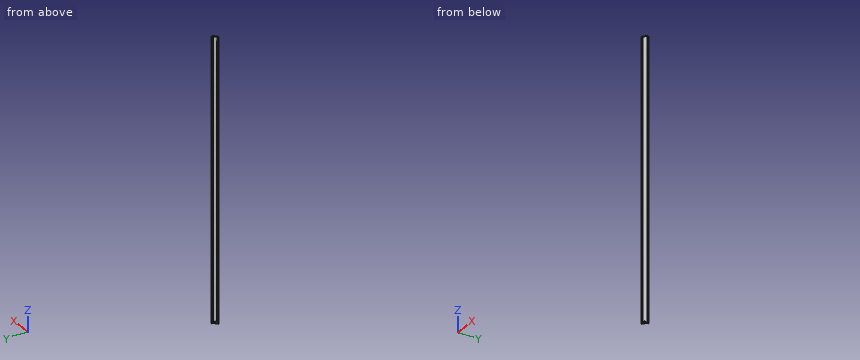
from build123d import *

# Parameters (mm, degrees)
F1_DEPTH = 28
F3_DEPTH = 2653
F5_DEPTH = 28
F6_R     = 2
F7_R     = 1
F8_R     = 4.25
F9_DEPTH = 25


with BuildPart() as f1:
    # F0 (on Top) → F1 (new body)
    with BuildSketch(Plane.XY):
        Polygon((-19.75, -17.750001), (-19.75, -19.75), (-9.25, -19.75), (19.75, 9.25), (19.75, 19.75), (17.750001, 19.75), (17.750001, 10.078427), (-10.078427, -17.750001), align=None)
    extrude(amount=F1_DEPTH)

    # F2 (on face) → F3 (join)
    with BuildSketch(Plane.XY.offset(28)):
        Polygon((-19.75, -19.75), (-9.25, -19.75), (19.75, 9.25), (19.75, 19.75), (11.25, 19.75), (11.25, 24.25), (9.25, 26.25), (9.25, 23.421573), (9.25, 19.75), (9.25, 17.750001), (17.750001, 17.750001), (17.750001, 10.078427), (16.585787, 8.914213), (-8.914213, -16.585787), (-10.078427, -17.750001), (-17.750001, -17.750001), (-17.750001, -9.25), (-19.75, -9.25), (-23.421573, -9.25), (-26.25, -9.25), (-24.25, -11.25), (-19.75, -11.25), align=None)
    extrude(amount=F3_DEPTH)

    # F4 (on face) → F5 (join)
    with BuildSketch(Plane.XY.offset(2681)):
        Polygon((19.75, 9.25), (19.75, 19.75), (17.750001, 19.75), (17.750001, 10.078427), (-10.078427, -17.750001), (-19.75, -17.750001), (-19.75, -19.75), (-9.25, -19.75), align=None)
    extrude(amount=F5_DEPTH)

    # F6
    f6_edges = [f1.edges().sort_by_distance(p)[0] for p in [
        (19.75, 9.25, 1354.5),
        (-9.25, -19.75, 1354.5),
    ]]
    fillet(f6_edges, radius=F6_R)

    # F7
    f7_edges = [f1.edges().sort_by_distance(p)[0] for p in [
        (-19.75, -19.75, 1354.5),
        (19.75, 19.75, 1354.5),
    ]]
    fillet(f7_edges, radius=F7_R)

    # F8 (on face) → F9 (cut)
    with BuildSketch(Plane(origin=(3.835787, -3.835787, 0), x_dir=(-0.707107, -0.707107, 0), z_dir=(-0.707107, 0.707107, 0))):
        with Locations((0, 14)):
            Circle(F8_R)
    extrude(amount=-F9_DEPTH, mode=Mode.SUBTRACT)


solid = f1.part
Part model, mm, in its own coordinate system. Round coordinates to 2 decimals unless told otherwise and drop trailing zeros. Write each loop counter-clockwise with the first axis right and the second up, starting at its lowest first coordinate (ties: lowest second). Pieces come first, ordered by that corner, then holes. Notation, with made-up numbers: M 66,52 L 92,52 A20 ccw 92,66 Z; hole C 26,20 d10. An arc over 180 degrees is marked long. Return JSON: item names as keys, results as strings. Group by question number.
(1) Drill centre lines: probe 1 along Y at (x, z) = (-10, 491); probe 2 along X at (y, z) = (13.5, 2329.5); probe 3 along Y at (x, z) = (-12.5, 894). Where is each one in solid material? Low to high.
(2) Pin check, flat tips, straight feed: pin 1 Ø4.5 at (y, z) = (-13.5, 1305) entering from +X; pin 2 Ø2.5 at (y, z) = (23.5, 1843.5) entering from -X; pin 3 Ø4 at (x, z) = (-20, 1991) entering from +Y; pin 4 Ø12 at (x, y) = (-12, -12.5) entering from -Z. Stop position of each tip, or through.
(3) Saw through at A-A on z = 2423.5. Write the cut outline in (x, y).
Returned:
{
 "1": {"probe 1": "-19.75 to -17.67", "probe 2": "17.75 to 19.75", "probe 3": "-19.75 to -17.75"},
 "2": {"pin 1": "x = -0.75", "pin 2": "x = 9.25", "pin 3": "y = -9.25", "pin 4": "z = 0"},
 "3": {"outline": "M -26.25,-9.25 L -24.25,-11.25 L -19.75,-11.25 L -19.75,-18.75 A1 ccw -18.75,-19.75 L -10.08,-19.75 A2 ccw -8.66,-19.16 L 19.16,8.66 A2 ccw 19.75,10.08 L 19.75,18.75 A1 ccw 18.75,19.75 L 11.25,19.75 L 11.25,24.25 L 9.25,26.25 L 9.25,17.75 L 17.75,17.75 L 17.75,10.08 L -10.08,-17.75 L -17.75,-17.75 L -17.75,-9.25 Z"}
}
